from build123d import *

# Parameters (mm, degrees)
SKETCH_W        = 10
SKETCH_H        = 5.5
PAD_DEPTH       = 3
SKETCH001_R     = 1.1
POCKET_DEPTH    = 3.001
SKETCH002_W     = 0.6
SKETCH002_H     = 0.6
POCKET001_DEPTH = 5.501
FILLET_R        = 0.75
CHAMFER_SIZE    = 1.2
CHAMFER001_SIZE = 0.4


with BuildPart() as part:
    # Sketch → Pad (new body)
    with BuildSketch(Plane.XY):
        with Locations((-5, 0)):
            Rectangle(SKETCH_W, SKETCH_H)
    extrude(amount=PAD_DEPTH)

    # Sketch001 (on Face6 of Pad) → Pocket (cut, through all)
    with BuildSketch(Plane.XY.offset(3)):
        with Locations((-6, 0)):
            Circle(SKETCH001_R)
    extrude(amount=-POCKET_DEPTH, mode=Mode.SUBTRACT)

    # Sketch002 (on Face1 of Pocket) → Pocket001 (cut, through all)
    with BuildSketch(Plane.XZ.offset(2.75)):
        with Locations((-8, 1.5)):
            Rectangle(SKETCH002_W, SKETCH002_H)
    extrude(amount=-POCKET001_DEPTH, mode=Mode.SUBTRACT)

    # Fillet
    fillet_edges = [part.edges().sort_by_distance(p)[0] for p in [
        (-10, -2.75, 1.5),
        (-10, 2.75, 1.5),
    ]]
    fillet(fillet_edges, radius=FILLET_R)

    # Mirrored: part across YZ


with BuildPart() as part_1:
    add(part.part)
    add(part.part.mirror(Plane.YZ))

    # Chamfer
    chamfer_edges = [part_1.edges().sort_by_distance(p)[0] for p in [
        (-7.1, 0, 3),
        (7.1, 0, 3),
    ]]
    chamfer(chamfer_edges, length=CHAMFER_SIZE)

    # Chamfer001
    chamfer001_edges = [part_1.edges().sort_by_distance(p)[0] for p in [
        (0, -2.75, 0),
    ]]
    chamfer(chamfer001_edges, length=CHAMFER001_SIZE)


solid = part_1.part
Design review of the part built by this model. Coordinates are the model's own, in mm. Round coordinates to 2 decimals unless told otherwise and drop trailing zeros. Write each loop counter-clockwise with the first axis right and the second up, starting at its lowest first coordinate (ties: lowest second). Pieces come first, ordered by that corner, then holes. Notation, with made-up numbers: (34, 47) -> (89, 47) arc R13 cw to (89, 55) -> close; hole circle Ø11 at (-7.5, 55.25). An arc over 180 degrees is marked (long way). One line per item, written item: value. Start each with the question number.
Q1. Add section B-B (y = 0). Give the boundary of the cut face in (x, z).
Q2. Add section C-C (x = 6). Give the boundary of the cut face in (y, z).
Q3. Add section D-D (z = 2.8). Give the boundary of the cut face in (x, y).
Q4. The part is to be moulded in two halves that separate along X. For faces 1 (the face through (-4.984, -0.421, 0.913)), 2 (the face through (0, -2.75, 2)), 3 (the face through (-10, 0, 2)), say which applies: pulls with the +X half, pulls with the -X half, needs draft (parallel to the pull), parting line crosses it, or undercut.
Q5. To check wall thickness, follow probe 1 along X at (y, z) = (-1.75, 1.4); probe 2 along Y at (x, z) = (6, 1.2); probe 3 along Z at (x, y) = (-8.25, 0.55). State the ranges of each line that lie inside material, in increasing order.
Q6. Add section A-A (z = 1.4). Give the boundary of the cut face in (x, y).
Response:
1. outline: (-10, 0.4) -> (-9.6, 0) -> (-7.1, 0) -> (-7.1, 1.8) -> (-8.3, 3) -> (-10, 3) -> close; (-4.9, 0) -> (4.9, 0) -> (4.9, 1.8) -> (3.7, 3) -> (-3.7, 3) -> (-4.9, 1.8) -> close; (7.1, 0) -> (9.6, 0) -> (10, 0.4) -> (10, 3) -> (8.3, 3) -> (7.1, 1.8) -> close; hole (-8.3, 1.2) -> (-7.7, 1.2) -> (-7.7, 1.8) -> (-8.3, 1.8) -> close; hole (7.7, 1.2) -> (8.3, 1.2) -> (8.3, 1.8) -> (7.7, 1.8) -> close
2. outline: (-2.75, 0.4) -> (-2.35, 0) -> (-1.1, 0) -> (-1.1, 1.8) -> (-2.3, 3) -> (-2.75, 3) -> close; (1.1, 0) -> (2.35, 0) -> (2.75, 0.4) -> (2.75, 3) -> (2.3, 3) -> (1.1, 1.8) -> close
3. outline: (-10, -2) arc R0.75 ccw to (-9.25, -2.75) -> (9.25, -2.75) arc R0.75 ccw to (10, -2) -> (10, 2) arc R0.75 ccw to (9.25, 2.75) -> (-9.25, 2.75) arc R0.75 ccw to (-10, 2) -> close; hole circle Ø4.2 at (-6, 0); hole circle Ø4.2 at (6, 0)
4. face 1: undercut
4. face 2: needs draft
4. face 3: pulls with the -X half
5. probe 1: x = -10 to -8.3, -7.7 to 7.7, 8.3 to 10
5. probe 2: y = -2.75 to -1.1, 1.1 to 2.75
5. probe 3: z = 0 to 1.2, 1.8 to 3
6. outline: (-10, -2) arc R0.75 ccw to (-9.25, -2.75) -> (-8.3, -2.75) -> (-8.3, 2.75) -> (-9.25, 2.75) arc R0.75 ccw to (-10, 2) -> close; (-7.7, -2.75) -> (7.7, -2.75) -> (7.7, 2.75) -> (-7.7, 2.75) -> close; (8.3, -2.75) -> (9.25, -2.75) arc R0.75 ccw to (10, -2) -> (10, 2) arc R0.75 ccw to (9.25, 2.75) -> (8.3, 2.75) -> close; hole circle Ø2.2 at (-6, 0); hole circle Ø2.2 at (6, 0)
